Input: part model. Units: mm. Frame: model coordinates. A direction names the side the tool comes from. Round coordinates to 2 decimals unless told otherwise and drop trailing zeros. Loops run counter-clockwise (first coordinate to the right, second up) from the corner with the lowest first, then second, coordinate; pieces in that order, holes last. Notation, with made-up numbers: (8, 8.25) - (48, 8.25) arc R22 cw to (48, 39.25) - close; hole circle Ø1 at (17, 20). An arc over 180 degrees is marked (long way). One line per question, with ' | ' between items. Start each with the question number.
Solid Edge part; units mm, degrees
sketch "Sketch1" plane through (0, 0, 0) normal (0, 0, 1) x (1, 0, 0)
  line L0 (-18, -6) -> (-15, -6)
  line L1 (-15, -6) -> (-15, 0)
  line L2 (-15, 0) -> (15, 0)
  line L3 (15, 0) -> (15, -6)
  line L4 (15, -6) -> (18, -6)
  line L5 (18, -6) -> (18, 3)
  line L6 (18, 3) -> (8, 3)
  line L7 (8, 3) -> (8, 11)
  line L8 (8, 11) -> (-8, 11)
  line L9 (-8, 11) -> (-8, 3)
  line L10 (-8, 3) -> (-18, 3)
  line L11 (-18, 3) -> (-18, -6)
  dimension "D1" = 18
  dimension "D2" = 15
  dimension "D3" = 8
  dimension "D4" = 15
  dimension "D5" = 8
extrude "Protrusion1" add sketch "Sketch1" along normal mid plane 5
sketch "Sketch2" plane through (0, 4.5, 2.5) normal (0, 0, 1) x (0, 1, 0)
  line L0 (-2, -5.5) -> (4, -5.5)
  line L1 (4, -5.5) -> (4, 5.5)
  line L2 (4, 5.5) -> (-2, 5.5)
  line L3 (-2, 5.5) -> (-2, -5.5)
  dimension "D1" = 4
extrude "Cutout1" cut sketch "Sketch2" against normal up to next
fillet "main_rounds" radius 2 10 edges at (8, 3, 0) (8, 11, 0) (5.5, 2.5, 0) (5.5, 8.5, 0) (-5.5, 8.5, 0) (-5.5, 2.5, 0) (-8, 3, 0) (-8, 11, 0) (-18, 3, 0) (18, 3, 0)
properties material "Polyethylene, low density"
(1) Reachability of faces 4 (the face through (-15, -3, 0)), 5 (the face through (-4.93, 7.9, -0.04)), 6 (the face through (8, 7, 0)) from +Z, -Z, +X, -X, +Y, -Y: full face, straight path, thin tool, end or side. Return the list, or none.
(2) Section A-A, the plane z = -0.9. Output: boundary loops of the cut face in (x, y), plus the area to 3 significant figures.
(3) Pin query (flat end, axial travel): P1, Ø1.2, axis at y = 8, z = -1, coming from the +X side; P2, Ø1, axis at x = -9, z = 0, coming from the -Y side; P3, Ø2, axis at y = 5.5, z = 0.5, coming from the +X side. Return the tip coordinate at first contact, or that it passes through.
(4) Line query: line 1 along X through (y, z) = (-1.5, 0.25); line 2 along Y through (x, z) = (-0.5, 2.05); line 3 along X through (y, z) = (2.75, 0.7). Output: solid intervals per line, ascending. Write a range as from..to.
(5) Section B-B, the plane x = 2. Output: boundary loops of the cut face in (y, z).
(6) Section D-D, the plane x = -13. Output: boundary loops of the cut face in (y, z), plus the area to 3 significant figures.
(7) Pull-direction query (Y, two-part tool) for faces 1 (the face through (0, 0, 0)), 2 (the face through (7.43, 10.4, 0.04)), 3 (the face through (5.5, 5, 0)); classes: released by +Y, released by -Y, zero draft, split by the parting line, or undercut.
(8) Section C-C, the plane y = -3. Output: boundary loops of the cut face in (x, z), plus the area to 3 significant figures.
Derived:
1) face 4: +Z, -Z, -Y | face 5: +Z, -Z | face 6: +Z, -Z, +X, +Y
2) outline: (-18, -6) - (-15, -6) - (-15, 0) - (15, 0) - (15, -6) - (18, -6) - (18, 1) arc R2 ccw to (16, 3) - (10, 3) arc R2 cw to (8, 5) - (8, 9) arc R2 ccw to (6, 11) - (-6, 11) arc R2 ccw to (-8, 9) - (-8, 5) arc R2 cw to (-10, 3) - (-16, 3) arc R2 ccw to (-18, 1) - close; hole (-5.5, 4.5) arc R2 ccw to (-3.5, 2.5) - (3.5, 2.5) arc R2 ccw to (5.5, 4.5) - (5.5, 6.5) arc R2 ccw to (3.5, 8.5) - (-3.5, 8.5) arc R2 ccw to (-5.5, 6.5) - close | area: 208 mm²
3) P1: stops at x = 8 | P2: stops at y = 0 | P3: stops at x = 8.06
4) line 1: x = -18..-15, 15..18 | line 2: y = 0..2.5, 8.5..11 | line 3: x = -16.97..-4.47, 4.47..16.97
5) outline: (0, -2.5) - (2.5, -2.5) - (2.5, 2.5) - (0, 2.5) - close; (8.5, -2.5) - (11, -2.5) - (11, 2.5) - (8.5, 2.5) - close
6) outline: (0, -2.5) - (3, -2.5) - (3, 2.5) - (0, 2.5) - close | area: 15.0 mm²
7) face 1: released by -Y | face 2: released by +Y | face 3: undercut
8) outline: (-18, -2.5) - (-15, -2.5) - (-15, 2.5) - (-18, 2.5) - close; (15, -2.5) - (18, -2.5) - (18, 2.5) - (15, 2.5) - close | area: 30.0 mm²
